```python
from build123d import *

# Parameters (mm, degrees)
SZKIC1_R                    = 5.45
DODANIE_WYCI_GNI_CIE1_DEPTH = 1.3
DODANIE_WYCI_GNI_CIE2_DEPTH = 2
SFAZOWANIE1_SIZE            = 0.4


with BuildPart() as part:
    # Szkic1 → Dodanie-wyciągnięcie1 (new body)
    with BuildSketch(Plane(origin=(0, 0, 0), x_dir=(1, 0, 0), z_dir=(0, 1, 0))):
        with Locations(Location((0, 0, 0), (0, 0, 270))):
            Circle(SZKIC1_R)
    extrude(amount=DODANIE_WYCI_GNI_CIE1_DEPTH)

    # Szkic2 → Dodanie-wyciągnięcie2 (add)
    with BuildSketch(Plane(origin=(0, 1.3, 0), x_dir=(1, 0, 0), z_dir=(0, 1, 0))):
        Polygon((2.280533563, 0), (1.140266782, 1.975), (-1.140266782, 1.975), (-2.280533563, 0), (-1.140266782, -1.975), (1.140266782, -1.975), align=None)
    extrude(amount=DODANIE_WYCI_GNI_CIE2_DEPTH)

    # Sfazowanie1
    sfazowanie1_edges = [part.edges().sort_by_distance(p)[0] for p in [
        (1.710400172, 3.3, 0.9875),
        (1.710400172, 3.3, -0.9875),
        (0, 3.3, -1.975),
        (-1.710400172, 3.3, -0.9875),
        (-1.710400172, 3.3, 0.9875),
        (0, 3.3, 1.975),
        (0, 1.3, -5.45),
    ]]
    chamfer(sfazowanie1_edges, length=SFAZOWANIE1_SIZE)


solid = part.part
```
Here's how the part is built. I have some questions about the finished solid (model axes, mm). A direction names the side the tool comes from. Give positions to 0.01 mm unless a question says otherwise; leave off trailing zeros. Write each loop counter-clockwise with the first axis right and the second up, starting at its lowest first coordinate (ties: lowest second). Pieces come first, ordered by that corner, then holes. Notation, with made-up numbers: (74.25, 52) -> (116.25, 52) arc R31 cw to (116.25, 80) -> close; hole circle Ø10 at (61.25, 83.25). An arc over 180 degrees is marked (long way). Use one line per item in the form item = value.
1) I'm going to push flat-ended pins straight in: pin 1 (0.8 mm diameter, centred on x = -0.5, y = 2, fed in from +Z) (3 decimals); pin 2 (1.5 mm diameter, centred on x = -3.5, y = 1.5, fed in from -Z); pin 3 (1.8 mm diameter, centred on x = 0.5, y = 2.5, fed in from -Z) (3 decimals). Where does each tip first touch, or does it pass through?
Verdict:
pin_1 = 1.975
pin_2 = -4.52
pin_3 = -1.975
2) On a 3-axis mill with a long thin cutter (end or side, diameter ignored), from which of +Z, -Z, +X, -X, +Y, -Y can I reach the whole of each face in a straight line? I mean faces 1 (the face through (-1.72, 2.09, 0.97)), 2 (the face through (-1.702, 2.089, -1.001)), 3 (the face through (0.1, 1.3, 2.2)). Say none if no direction works.
Verdict:
face_1 = +Z, -X, +Y
face_2 = -Z, -X, +Y
face_3 = +Y
3) Suppose I cut it at A-A (x = 0). Please give me the cut outline in (y, z) (3 decimals).
Verdict:
outline = (0, -5.45) -> (0.9, -5.45) -> (1.3, -5.05) -> (1.3, -1.975) -> (2.9, -1.975) -> (3.3, -1.575) -> (3.3, 1.575) -> (2.9, 1.975) -> (1.3, 1.975) -> (1.3, 5.05) -> (0.9, 5.45) -> (0, 5.45) -> close
4) If I drill on L1, parallel to Y at x = -1.75, z = 3.75; L2, parallel to Z at x = 0.5, y = 1.4 (3 decimals); L3, parallel to X at y = 0.6, z = 0.25, over which ranges is the centre line in solid material (lowest first)? Write a range as [from, to].
Verdict:
L1 = [0, 1.3]
L2 = [-1.975, 1.975]
L3 = [-5.44, 5.44]
5) Suppose I cut it at B-B (y = 1.7). Please give me the cut outline in (x, z) (3 decimals), and give its area (3 significant figures).
Verdict:
outline = (-2.281, 0) -> (-1.14, -1.975) -> (1.14, -1.975) -> (2.281, 0) -> (1.14, 1.975) -> (-1.14, 1.975) -> close
area = 13.5 mm2
